Check sheet for the modelled part. Datum: model origin and axes. Units: mm. Face numbers are marked on the shaded views. A direction names the side the tool comes from. Round coordinates to 2 decimals unless told otherwise and drop trailing zeros. Order: outer loops, then holes, each group sorted by start corner. A loop starts at its lowest first (then second) coordinate and runs counter-clockwise, first axis right, second up.
```python
from build123d import *

# Parameters (mm, degrees)
F3_DEPTH   = 3.09
F7_DEPTH   = 12.02
F8_R       = 0.98
F9_DEPTH   = 20.601
F8_R_2     = 2.925
F10_DEPTH  = 2.17
F10_FACE_R = 2.925
F11_DEPTH  = 19.62
F12_R      = 1.385
F13_DEPTH  = 1.12
F15_DEPTH  = 4.13


with BuildPart() as f1:
    # F0 (on Front) → F1 (revolve)
    with BuildSketch(Plane.XZ):
        Polygon((0, -73.89), (0, -7.79), (-4.325, -7.79), (-4.325, 0), (-7.97, 0), (-7.97, -3.67), (-6, -3.67), (-6, -11.4), (-7.97, -11.4), (-7.97, -14.31), (-4.66, -14.31), (-4.66, -15.65), (-7.97, -15.65), (-7.97, -16.87), (-4.66, -16.87), (-4.66, -18.21), (-12.5, -18.21), (-12.5, -19.43), (-4.66, -19.43), (-4.66, -21.605556), (-12.5, -21.605556), (-12.5, -22.825556), (-4.66, -22.825556), (-4.66, -25.001111), (-12.5, -25.001111), (-12.5, -26.221111), (-4.66, -26.221111), (-4.66, -28.396667), (-12.5, -28.396667), (-12.5, -29.616667), (-4.66, -29.616667), (-4.66, -31.792222), (-12.5, -31.792222), (-12.5, -33.012222), (-4.66, -33.012222), (-4.66, -35.187778), (-12.5, -35.187778), (-12.5, -36.407778), (-6.52, -36.407778), (-6.52, -38.583333), (-12.5, -38.583333), (-12.5, -39.803333), (-6.52, -39.803333), (-6.52, -41.978889), (-12.5, -41.978889), (-12.5, -43.198889), (-6.52, -43.198889), (-6.52, -45.374444), (-12.5, -45.374444), (-12.5, -46.594444), (-6.52, -46.594444), (-6.52, -48.77), (-12.5, -48.77), (-12.5, -49.99), (-2.94, -49.99), (-2.94, -71.96), (-2.305, -71.96), (-0.3475, -73.89), align=None)
    revolve(axis=Axis((0, 0, -36.945), (0, 0, -1)))

    # F2 (on face) → F3 (join)
    with BuildSketch(Plane(origin=(0, 0, -71.96), x_dir=(1, 0, 0), z_dir=(0, 0, -1))):
        Polygon((-4.085, 2.358476), (-4.085, -2.358476), (0, -4.716952), (4.085, -2.358476), (4.085, 2.358476), (0, 4.716952), align=None)
    extrude(amount=-F3_DEPTH)

    # F4 (on Front) → F5 (revolve, cut)
    with BuildSketch(Plane.XZ):
        Polygon((-4.085, -72.96), (-4.085, -71.96), (-5.63, -70.415), (-4.085, -68.87), (-4.085, -67.87), (-7.085, -67.87), (-7.085, -72.96), align=None)
    revolve(axis=Axis((0, 0, -72.455682), (0, 0, -1)), mode=Mode.SUBTRACT)

    # F6 (on face) → F7 (join)
    with BuildSketch(Plane.XY.offset(-68.87)):
        Polygon((-8.1, -11.04), (0, -11.04), (8.1, -11.04), (8.1, 4.98), (0, 4.98), (-8.1, 4.98), align=None)
    extrude(amount=F7_DEPTH)

    # F8 (on face) → F9 (cut, through all)
    with BuildSketch(Plane(origin=(-8.1, 0, 0), x_dir=(0, -1, 0), z_dir=(-1, 0, 0))):
        with Locations((8.79, -58.94)):
            Circle(F8_R)
    extrude(amount=-F9_DEPTH, mode=Mode.SUBTRACT)

    # F8 (on face) → F10 (join)
    with BuildSketch(Plane(origin=(-8.1, 0, 0), x_dir=(0, -1, 0), z_dir=(-1, 0, 0))):
        with Locations((6.655, -63.875)):
            Circle(F8_R_2)
    extrude(amount=F10_DEPTH)

    # F10_face (on face) → F11 (join)
    with BuildSketch(Plane(origin=(-10.27, -6.655, -63.875), x_dir=(0, -1, 0), z_dir=(-1, 0, 0))):
        Circle(F10_FACE_R)
    extrude(amount=-F11_DEPTH)

    # F12 (on face) → F13 (join)
    with BuildSketch(Plane(origin=(0, 0, -68.87), x_dir=(1, 0, 0), z_dir=(0, 0, -1))):
        with Locations((0, 7.085)):
            Circle(F12_R)
    extrude(amount=F13_DEPTH)

    # F14 (on face) → F15 (join)
    with BuildSketch(Plane(origin=(0, 0, -49.99), x_dir=(1, 0, 0), z_dir=(0, 0, -1))):
        Polygon((2.777055, 4.81), (-2.777055, 4.81), (-5.55411, 0), (-2.777055, -4.81), (2.777055, -4.81), (5.55411, 0), align=None)
    extrude(amount=F15_DEPTH)

    # F16 (on Right) → F17 (revolve, cut)
    with BuildSketch(Plane.YZ):
        Polygon((6.875, -52.055), (4.81, -54.12), (8.81, -54.12), (8.81, -49.99), (4.81, -49.99), align=None)
    revolve(axis=Axis((0, 0, -29.465), (0, 0, -1)), mode=Mode.SUBTRACT)


solid = f1.part
```
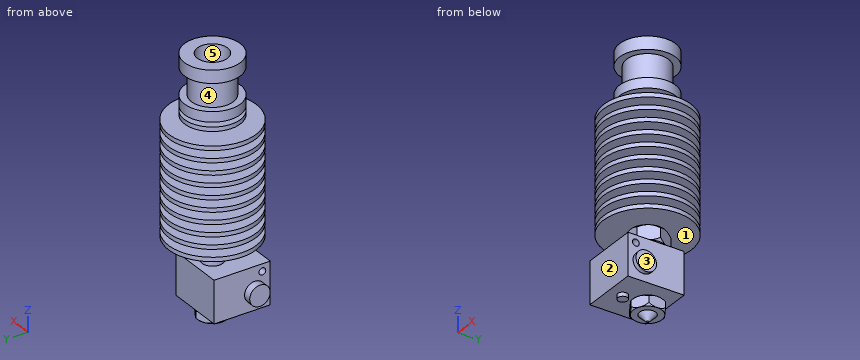
Item 1: Release check for a two-part mould opening along Z. For the marked faces 4 and 5 record: released by +Z, released by -Z, zero draft, split by the parting line, or undercut.
Answer:
face 4: undercut
face 5: zero draft
Item 2: Sectioned sample at C-C (y = 9.5). State how many separate pieces and enclosed holes the cut face has, and give its area (3 significant figures).
Answer:
separate pieces: 10
enclosed holes: 0
area: 198 mm2
Item 3: Go/stop test with flat-tipped pins: P1, Ø2, axis at y = 3.5, z = -49.5, coming from the -X side; P2, Ø7.5, axis at x = 2, y = 6, coming from the -Z side; P3, Ø1.5, axis at y = 0, z = -54, coming from the +X side. Record where each tip stops, or that it passes through.
Answer:
P1: stops at x = -12.25
P2: stops at z = -71.96
P3: stops at x = 5.55
Item 4: Sectioned sample at B-B (z = -9.5). Record the cut outline in (x, y).
Answer:
outline: circle Ø12 at (0, 0)
Item 5: Sectioned sample at A-A (z = -58.94). Record the cut outline in (x, y).
Answer:
outline: (-8.1, -11.04) - (8.1, -11.04) - (8.1, -9.77) - (-8.1, -9.77) - close; (-8.1, -7.81) - (8.1, -7.81) - (8.1, 4.98) - (-8.1, 4.98) - close
Item 6: Access from +Z, -Z, +X, -X, +Y, -Y to the whole of each face (thin tool, end or side, straight path). Record for the marked faces 1, 2 and 3.
Answer:
face 1: none
face 2: -Z, +X, -X, -Y
face 3: -Z, +X, +Y, -Y
Item 7: Scan lines: line 1 along Y through (x, z) = (0, -5.25) (3 decimals); line 2 along Y through (x, z) = (0, -2) (3 decimals); line 3 along X through (y, z) = (4.5, -44.5). Record each from-to range of solid material in increasing order.
Answer:
line 1: y = -6 to -4.325, 4.325 to 6
line 2: y = -7.97 to -4.325, 4.325 to 7.97
line 3: x = -4.72 to 4.72
